Input: part model. Units: mm. Frame: model coordinates. Face numbers are marked on the shaded views. A direction names the side the tool comes from. Coordinates: 2 decimals unless noted, no trailing zeros. Loops run counter-clockwise (first coordinate to the right, second up) from the corner with the lowest first, then second, coordinate; pieces in that order, holes last.
Item 1: Reachability of the marked faces 1, 2, 3 and 4 from +Z, -Z, +X, -X, +Y, -Y: full face, straight path, thin tool, end or side. Return the list, or none.
Item 2: Section A-A on x = 14.75. Return loops of the section in (y, z), and give its area (3 significant figures).
Item 3: Section D-D on z = -10.75. Return loops of the section in (x, y).
Item 4: Ray query, line 1 along X through (y, z) = (9.25, -5.75); line 2 along Z through (x, y) = (-0.25, 2); line 3 along X through (y, z) = (-7.75, 0.25). Return the intervals inside material, ascending.
Item 5: Section C-C on x = 2.25. Return loops of the section in (y, z).
Item 6: Section B-B on z = 10.25. Return loops of the section in (x, y), and give its area (3 significant figures).
Item 7: Contact query for flat-ended pins moving along their axis: P1, Ø12, axis at x = 12.5, y = -7.5, coming from the -Z side; P2, Ø4, axis at x = -3, y = 2.5, coming from the -Z side; P3, Ø2, axis at y = 9.5, z = 5, coming from the -X side. Output: stop coordinate, or through.
Item 8: Pull-direction query (X, two-part tool) for the marked faces 5, 6 and 7; classes: released by +X, released by -X, zero draft, split by the parting line, or undercut.
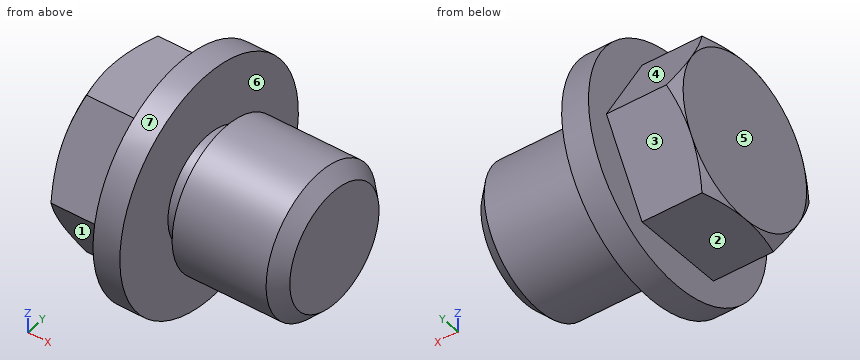
Autodesk Inventor part; units mm, degrees
ref_plane "工作平面2" through (0, 0, 0) normal (-1, 0, 0) x (0, 0, 1)
ref_plane "Work Plane1" through (1.525, 0, 0) normal (0, 0, 1) x (1, 0, 0)
ref_plane "YZ Plane" through (0, 0, 0) normal (1, 0, 0) x (0, 1, 0)
sketch "草图1" plane through (0, 0, 0) normal (0, 0, 1) x (1, 0, 0)
  line L0 (0, 6) -> (45, 6)
  line L1 (45, 6) -> (45, 0)
  line L2 (45, 0) -> (0, 0)
  line L3 (-9, 0) -> (54, 0)
  line L4 (0, -1.2) -> (0, 7.2)
  line L5 (0, 6) -> (0, 0)
  dimension "d2" = 12
  dimension "d59" = 45
ref_plane "工作平面2" through (0, 0, 0) normal (-1, 0, 0) x (0, 0, 1)
sketch "草图2" plane through (0, 0, 0) normal (-1, 0, 0) x (0, 0, 1)
  line L0 (0, 10.3923) -> (9, 5.1962)
  line L1 (9, 5.1962) -> (9, -5.1962)
  line L2 (9, -5.1962) -> (0, -10.3923)
  line L3 (0, -10.3923) -> (-9, -5.1962)
  line L4 (-9, -5.1962) -> (-9, 5.1962)
  line L5 (-9, 5.1962) -> (0, 10.3923)
  line L6 (-12.6, 0) -> (12.6, 0)
  line L7 (0, 14.5492) -> (0, -14.5492)
  point P0 (0, 0)
  point P1 (0, 0)
  dimension "d11" = 18
extrude "头" add sketch "草图2" along normal blind 7.5
sketch "草图4" plane through (0, 0, 0) normal (0, 0, 1) x (1, 0, 0)
  line L0 (-6.4608, 10.8) -> (-7.5, 9)
  line L1 (-1.1, 0) -> (-0.234, 0)
  line L2 (-18, 0) -> (55.5, 0)
  line L3 (-7.5, 10.8) -> (-6.4608, 10.8)
  line L4 (-7.5, 9) -> (-7.5, 10.8)
  line L5 (0, 12.96) -> (0, -2.16)
  dimension "d65" = 18
  dimension "d67" = 30
  dimension "d68" = 21.6
  dimension "d69" = 7.5
revolve "倒角1" cut sketch "草图4" angle 360 about axis through (-1.1, 0, 0) along (1, 0, 0)
ref_plane "Work Plane1" through (1.525, 0, 0) normal (0, 0, 1) x (1, 0, 0)
sketch "草图7" plane through (0, 0, 0) normal (1, 0, 0) x (0, 0, -1)
  circle A0 centre (0, 0) radius 13
  dimension "d74" = 26
extrude "拉伸5" add sketch "草图7" along normal blind 3
sketch "草图8" plane through (3, 0, 0) normal (1, 0, 0) x (0, 0, -1)
  circle A0 centre (0, 0) radius 13
  circle A1 centre (0, 0) radius 6
  dimension "d77" = 12
extrude "拉伸6" add sketch "草图8" along normal blind 2 contours A1
sketch "草图9" plane through (5, 0, 0) normal (1, 0, 0) x (0, 0, -1)
  circle A0 centre (0, 0) radius 8
  dimension "d80" = 16
extrude "拉伸7" add sketch "草图9" along normal blind 12
chamfer "倒角2" distance 1.5 angle 45 1 edges at (17, 0, 8)
thread "螺纹3"
equation "\"d2\" = GD"
equation "\"d59\" = NLG"
equation "\"d11\" = SW"
equation "\"d3\" = KOH"
equation "\"d65\" = SW"
equation "\"d67\" = ANG1"
equation "\"d68\" = 1.2 * SW"
equation "\"d69\" = KOH"
equation "\"NLG\" = 45"
equation "\"GD\" = NND"
equation "\"BDM\" = NND"
equation "\"KOH\" = 7.5"
equation "\"SW\" = 18"
equation "\"SW0\" = SW"
equation "\"SPD\" = NND - 1.2269 * PTC"
equation "\"SD2\" = NND"
equation "\"SD\" = 0"
equation "\"ANG1\" = 30deg"
equation "\"GAL\" = 0.61345 * PTC"
equation "\"GUL\" = 0.61345 * PTC"
equation "\"RR\" = 0.6"
equation "\"RR1\" = 0.1"
equation "\"WFT\" = 0"
equation "\"GD1\" = THREADDIA - 1.2269 * PTC"
equation "\"THREADDIA\" = 12"
equation "\"SDH\" = SW"
equation "\"TOA\" = 30deg"
equation "\"FAWI\" = 90deg"
equation "\"PTC\" = 1.75"
equation "\"NND\" = 12"
equation "\"E0\" = 1.155 * SW"
properties part number "六角螺栓 GB/T 5780 M12 x 45" material "钢，软"
Results found:
1. face 1: -Z, -X, -Y
1. face 2: -Z, -X, +Y, -Y
1. face 3: -Z, -X, +Y
1. face 4: +Z, -X, +Y
2. outline: circle Ø16 at (0, 0)
2. area: 201 mm2
3. outline: (0, -7.31) - (3, -7.31) - (3, 7.31) - (0, 7.31) - close
4. line 1: x = 0 to 3
4. line 2: z = -9 to 9
4. line 3: x = -7.5 to 3, 5 to 15.75
5. outline: circle Ø26 at (0, 0)
6. outline: (0, -8) - (3, -8) - (3, 8) - (0, 8) - close
6. area: 48.0 mm2
7. P1: stops at z = -7.86
7. P2: stops at z = -9
7. P3: stops at x = 0
8. face 5: released by -X
8. face 6: undercut
8. face 7: zero draft
